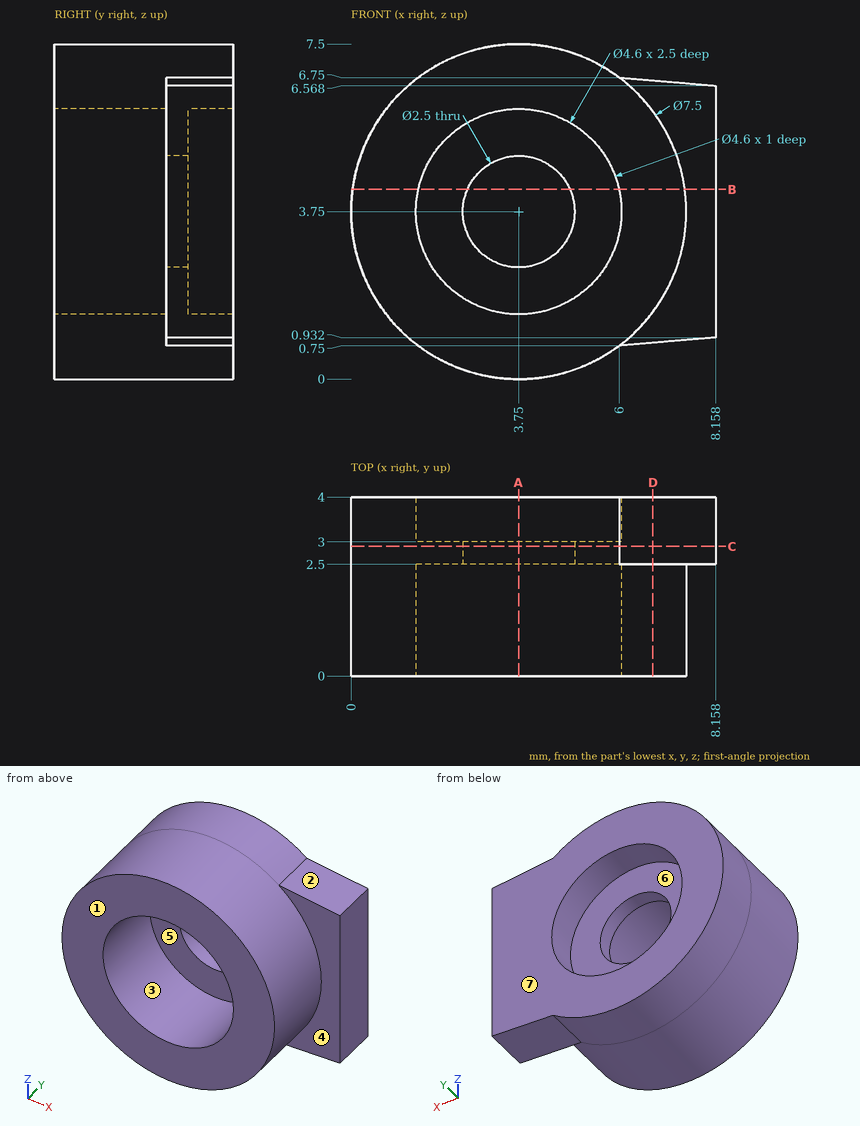
Study the drawing (mm; zero at the part's minimum x, y, z) and answer. A direction names the side the tool comes from. Coordinates: 2 decimals unless noted, no trailing zeros. Write each loop counter-clockwise with the first axis right and the second up, starting at its lowest first coordinate (ties: lowest second). Pieces come first, ordered by that corner, then holes. Notation, with made-up numbers: (-14, 55.25) - (14, 55.25) arc R24 cw to (14, 73.25) - close; hole circle Ø9 at (-22.75, -22.5). An arc over 180 degrees is marked (long way). Answer as a JSON object with one key per item and string values. Group by question number.
1. Consider L1, parallel to X at y = 2.8, z = 3.75; L2, parallel to X at y = 3.7, z = 3.75; L3, parallel to Z at x = 3.75, y = 1.2. Determine where each line is inside the solid, lowest interval first. Write a range as [from, to].
2. A cutting plane is placed at B-B (z = 4.25). Determine the outline of the cut face in (x, y) (1 decimal), plus the area to 3 significant figures.
3. Which of the six approach directions +Z, -Z, +X, -X, +Y, -Y give full straight-line access (tool end or side, diameter ignored) to the marked faces 4, 5, 6 and 7?
4. A cutting plane is placed at C-C (y = 2.9). Determine the outline of the cut face in (x, z).
5. Each of these flat-tipped pins is pushed along its axis until it touches: P1, Ø1, axis at x = 3, y = 2, coming from the -Z side; P2, Ø1.5, axis at x = 3.75, z = 3.75, coming from the -Y side; P3, Ø4, axis at x = 3.75, z = 3.75, coming from the -Y side; P4, Ø2, axis at y = 2.5, z = 5.5, coming from the -X side. Where does it stop, or does it pass through?
6. The mould has two halves that part along X. Classify the marked faces 1, 2 and 3: +X half, -X half, draft (parallel to the pull), parting line (faces both ways), or undercut.
7. A cutting plane is placed at A-A (x = 3.75). Determine the outline of the cut face in (y, z).
8. A cutting plane is placed at D-D (x = 6.75). Determine the outline of the cut face in (y, z).
Worked out:
{
 "1": {"L1": "x = [0, 2.5], [5, 8.16]", "L2": "x = [0, 1.45], [6.05, 8.16]", "L3": "z = [0, 1.45], [6.05, 7.5]"},
 "2": {"outline": "(0, 0) - (1.5, 0) - (1.5, 2.5) - (2.6, 2.5) - (2.6, 3) - (1.5, 3) - (1.5, 4) - (0, 4) - close; (4.9, 2.5) - (6, 2.5) - (6, 0) - (7.5, 0) - (7.5, 2.5) - (8.2, 2.5) - (8.2, 4) - (6, 4) - (6, 3) - (4.9, 3) - close", "area": "13.9 mm²"},
 "3": {"face 4": "+X, -Y", "face 5": "-Y", "face 6": "+Y", "face 7": "+Z, -Z, +X, -X, +Y"},
 "4": {"outline": "(6, 0.75) - (8.16, 0.93) - (8.16, 6.57) - (6, 6.75) arc R3.75 ccw (long way) to start; hole circle Ø2.5 at (3.75, 3.75)"},
 "5": {"P1": "stops at z = 0.01", "P2": "passes through", "P3": "stops at y = 2.5", "P4": "stops at x = 0.08"},
 "6": {"face 1": "draft", "face 2": "+X half", "face 3": "undercut"},
 "7": {"outline": "(0, 0) - (4, 0) - (4, 1.45) - (3, 1.45) - (3, 2.5) - (2.5, 2.5) - (2.5, 1.45) - (0, 1.45) - close; (0, 6.05) - (2.5, 6.05) - (2.5, 5) - (3, 5) - (3, 6.05) - (4, 6.05) - (4, 7.5) - (0, 7.5) - close"},
 "8": {"outline": "(0, 1.5) - (2.5, 1.5) - (2.5, 0.81) - (4, 0.81) - (4, 6.69) - (2.5, 6.69) - (2.5, 6) - (0, 6) - close"}
}
